from build123d import *

# Parameters (mm, degrees)
F1_DEPTH = 101.6
F2_W     = 38.1
F2_H     = 38.1
F3_DEPTH = 25.4
F4_DEPTH = 25.4
F2_W_2   = 19.05
F2_H_2   = 50.8
F5_DEPTH = 25.4


with BuildPart() as f1:
    # F0 (on Top) → F1 (new body)
    with BuildSketch(Plane.XY):
        Polygon((1219.2, -9.525), (1219.2, 0), (1219.2, 9.525), (-1219.2, 9.525), (-1219.2, 0), (-1219.2, -9.525), align=None)
    extrude(amount=-F1_DEPTH)

    # F2 (on face) → F3 (cut)
    with BuildSketch(Plane.XZ.offset(9.525)):
        with Locations((590.55, -82.55)):
            Rectangle(F2_W, F2_H)
    extrude(amount=-F3_DEPTH, mode=Mode.SUBTRACT)

    # F2 (on face) → F4 (cut)
    with BuildSketch(Plane.XZ.offset(9.525)):
        with Locations((-590.55, -82.55)):
            Rectangle(F2_W, F2_H)
    extrude(amount=-F4_DEPTH, mode=Mode.SUBTRACT)

    # F2 (on face) → F5 (cut)
    with BuildSketch(Plane.XZ.offset(9.525)):
        with Locations((-904.875, -25.4)):
            Rectangle(F2_W_2, F2_H_2)
        Polygon((-452.4375, 0), (-461.9625, 0), (-461.9625, -50.8), (-442.9125, -50.8), (-442.9125, 0), align=None)
        Polygon((9.525, -50.8), (9.525, 0), (0, 0), (-9.525, 0), (-9.525, -50.8), (0, -50.8), align=None)
        Polygon((461.9625, -50.8), (461.9625, 0), (452.4375, 0), (442.9125, 0), (442.9125, -50.8), align=None)
        with Locations((904.875, -25.4)):
            Rectangle(F2_W_2, F2_H_2)
    extrude(amount=-F5_DEPTH, mode=Mode.SUBTRACT)


solid = f1.part
Could you check a few things on this model? Use its own coordinates, in mm. Give positions to 0.01 mm unless a question says otherwise; leave off trailing zeros.
1. For pin 1 (9.5 mm diameter, centred on x = -596.5, y = 2.5, fed in from -Z); pin 2 (9.5 mm diameter, centred on x = 0, y = 3.5, fed in from +Z); pin 3 (6 mm diameter, centred on x = 915.5, y = -1.5, fed in from +Z), each with a flat end and sliding along its axis, tell me the tip position at first contact or that it passes through.
Answers below:
pin 1: stops at z = -63.5
pin 2: stops at z = -50.8
pin 3: stops at z = 0
2. Suppose I cut it at A-A (z = -17.5). State how many separate pieces and enclosed holes the cut face has, plus the area to 3 significant figures.
Answers below:
separate pieces: 6
enclosed holes: 0
area: 44,600 mm2
3. I need wall thicknesses on L1, parallel to X at y = 5, z = -92; L2, parallel to Z at x = -579, y = -2; L3, parallel to Z at x = 902, y = -4. Which ranges of each line are inside material? Lowest first, please.
Answers below:
L1: x = -1219.2 to -609.6, -571.5 to 571.5, 609.6 to 1219.2
L2: z = -63.5 to 0
L3: z = -101.6 to -50.8
